Part model, mm, in its own coordinate system. A direction names the side the tool comes from. Give positions to 0.01 mm unless a question says otherwise; leave off trailing zeros. Answer in a Markdown table with one row per item.
from build123d import *

# Parameters (mm, degrees)
BOSS_EXTRUDE1_DEPTH           = 4.7625
SKETCH2_R                     = 4.7625
GEARBOX_WITH_PRESS_FITS_DEPTH = 412.602247496
SKETCH3_R                     = 1.58115
CUT_EXTRUDE1_DEPTH            = 412.602247496
F_4_CLEARANCE_HOLE2_D         = 3.2639
F_4_CLEARANCE_HOLE2_DEPTH     = 28.702
F_4_CLEARANCE_HOLE2_TIP       = 0.980574487
F_4_CLEARANCE_HOLE1_D         = 3.2639
F_4_CLEARANCE_HOLE1_DEPTH     = 4.826
F_4_CLEARANCE_HOLE1_TIP       = 0.980574487
CUT_EXTRUDE2_DEPTH            = 412.602247496


with BuildPart() as part:
    # Sketch1 → Boss-Extrude1 (new body)
    with BuildSketch(Plane(origin=(0, 0, 0), x_dir=(0, 0, -1), z_dir=(1, 0, 0))):
        Polygon((33.297595377, -40.64), (312.697595377, -40.64), (345.995190754, -12.7), (409.563327383, 40.64), (312.697595377, 40.64), (33.297595377, 40.64), (0, 12.7), (-63.568136629, -40.64), align=None)
    extrude(amount=BOSS_EXTRUDE1_DEPTH)

    # Sketch2 → Gearbox (with Press fits) (cut, through all)
    with BuildSketch(Plane(origin=(4.7625, 0, 0), x_dir=(0, 0, -1), z_dir=(1, 0, 0))):
        with Locations((331.004197306, 10)):
            Circle(SKETCH2_R)
    extrude(amount=-GEARBOX_WITH_PRESS_FITS_DEPTH, mode=Mode.SUBTRACT)

    # Sketch3 → Cut-Extrude1 (cut, through all)
    with BuildSketch(Plane(origin=(4.7625, 0, 0), x_dir=(0, 0, -1), z_dir=(1, 0, 0))):
        with Locations((287.297595377, 36.83)):
            Circle(SKETCH3_R)
        with Locations((230.147595377, 36.83)):
            Circle(SKETCH3_R)
        with Locations((172.997595377, 36.83)):
            Circle(SKETCH3_R)
        with Locations((115.847595377, 36.83)):
            Circle(SKETCH3_R)
        with Locations((58.697595377, 36.83)):
            Circle(SKETCH3_R)
        with Locations((58.697595377, -36.83)):
            Circle(SKETCH3_R)
        with Locations((115.847595377, -36.83)):
            Circle(SKETCH3_R)
        with Locations((172.997595377, -36.83)):
            Circle(SKETCH3_R)
        with Locations((230.147595377, -36.83)):
            Circle(SKETCH3_R)
        with Locations((287.297595377, -36.83)):
            Circle(SKETCH3_R)
    extrude(amount=-CUT_EXTRUDE1_DEPTH, mode=Mode.SUBTRACT)

    # #4 Clearance Hole2
    with Locations(Plane(origin=(4.7625, 0, 0), x_dir=(0, 0, -1), z_dir=(1, 0, 0))):
        with Locations((327.962613202, -22.8575274), (342.555759844, -10.612423436), (367.850547356, 10.612423436), (382.443693997, 22.8575274), (18.032577552, 22.8575274), (3.43943091, 10.612423436), (-21.855356602, -10.612423436), (-36.448503243, -22.8575274)):
            Hole(F_4_CLEARANCE_HOLE2_D / 2, depth=F_4_CLEARANCE_HOLE2_DEPTH)
            with Locations((0, 0, -(F_4_CLEARANCE_HOLE2_DEPTH + F_4_CLEARANCE_HOLE2_TIP / 2))):  # 118° drill point
                Cone(0, F_4_CLEARANCE_HOLE2_D / 2, F_4_CLEARANCE_HOLE2_TIP, mode=Mode.SUBTRACT)

    # #4 Clearance Hole1
    with Locations(Plane(origin=(4.7625, 0, 0), x_dir=(0, 0, -1), z_dir=(1, 0, 0))):
        with Locations((198.397595377, 35.56), (198.397595377, -35.56), (198.397595377, 0)):
            Hole(F_4_CLEARANCE_HOLE1_D / 2, depth=F_4_CLEARANCE_HOLE1_DEPTH)
            with Locations((0, 0, -(F_4_CLEARANCE_HOLE1_DEPTH + F_4_CLEARANCE_HOLE1_TIP / 2))):  # 118° drill point
                Cone(0, F_4_CLEARANCE_HOLE1_D / 2, F_4_CLEARANCE_HOLE1_TIP, mode=Mode.SUBTRACT)

    # Sketch11 → Cut-Extrude2 (cut, through all)
    with BuildSketch(Plane(origin=(4.7625, 0, 0), x_dir=(0, 0, -1), z_dir=(1, 0, 0))):
        with BuildLine():
            Line((-21.992783256, -22.332808893), (35.744876514, 26.114840125))
            ThreePointArc((35.744876514, 26.114840125), (37.885826828, 26.856070682), (39.975806034, 25.981383362))
            Line((39.975806034, 25.981383362), (90.827068404, -22.466265655))
            ThreePointArc((90.827068404, -22.466265655), (91.584794367, -25.944437039), (88.636989544, -27.94))
            Line((88.636989544, -27.94), (-19.951932595, -27.94))
            ThreePointArc((-19.951932595, -27.94), (-22.935456666, -25.850913955), (-21.992783256, -22.332808893))
        make_face()
        with BuildLine():
            Line((62.076755313, 22.466265655), (112.793727505, -25.853440749))
            ThreePointArc((112.793727505, -25.853440749), (114.983806365, -26.729706404), (117.173885225, -25.853440749))
            Line((117.173885225, -25.853440749), (167.890857417, 22.466265655))
            ThreePointArc((167.890857417, 22.466265655), (168.648583379, 25.944437039), (165.700778557, 27.94))
            Line((165.700778557, 27.94), (64.266834173, 27.94))
            ThreePointArc((64.266834173, 27.94), (61.31902935, 25.944437039), (62.076755313, 22.466265655))
        make_face()
        with BuildLine():
            Line((186.682516517, 22.828515143), (139.140544325, -22.466265655))
            ThreePointArc((139.140544325, -22.466265655), (138.382818363, -25.944437039), (141.330623185, -27.94))
            Line((141.330623185, -27.94), (188.872595377, -27.94))
            ThreePointArc((188.872595377, -27.94), (191.117659407, -27.01006403), (192.047595377, -24.765))
            Line((192.047595377, -24.765), (192.047595377, 20.529780798))
            ThreePointArc((192.047595377, 20.529780798), (190.123020229, 23.448181506), (186.682516517, 22.828515143))
        make_face()
        with BuildLine():
            Line((204.747595377, 18.932195541), (204.747595377, -24.765))
            ThreePointArc((204.747595377, -24.765), (205.677531347, -27.01006403), (207.922595377, -27.94))
            Line((207.922595377, -27.94), (243.096578394, -27.94))
            ThreePointArc((243.096578394, -27.94), (245.960282851, -26.13606593), (245.569855632, -22.774139707))
            Line((245.569855632, -22.774139707), (210.395872614, 20.923055835))
            ThreePointArc((210.395872614, 20.923055835), (206.867140553, 21.926630398), (204.747595377, 18.932195541))
        make_face()
        with BuildLine():
            Line((225.209113147, 22.774139707), (263.999518653, -25.415794703))
            ThreePointArc((263.999518653, -25.415794703), (266.163859962, -26.584868521), (268.513646551, -25.857125516))
            Line((268.513646551, -25.857125516), (325.94417401, 22.332808893))
            ThreePointArc((325.94417401, 22.332808893), (326.88684742, 25.850913955), (323.903323349, 27.94))
            Line((323.903323349, 27.94), (227.682390385, 27.94))
            ThreePointArc((227.682390385, 27.94), (224.818685928, 26.13606593), (225.209113147, 22.774139707))
        make_face()
    extrude(amount=-CUT_EXTRUDE2_DEPTH, mode=Mode.SUBTRACT)


solid = part.part
(1) Drill centre lines: line 1 along Y through (x, z) = (4.45, 21); line 2 along Y through (x, z) = (4.1, -38.5); line 3 along Y through (x, z) = (0.85, -116.5). Where is each one in solid material? Low to high.
Recorded:
| item | result |
|---|---|
| line 1 | y = -40.64 to -27.76, -21.5 to -12, -9.22 to -4.92 |
| line 2 | y = -40.64 to -27.94, 26.78 to 40.64 |
| line 3 | y = -40.64 to -38.27, -35.39 to -26.34, 27.94 to 35.39, 38.27 to 40.64 |
(2) Saw through at A-A (x = 2.5). Give the number of separate pieces and of enclosed holes in the cut face, plus the area to 3 significant figures.
Recorded:
| item | result |
|---|---|
| separate pieces | 1 |
| enclosed holes | 27 |
| area | 17,700 mm^2 |
(3) Pull direction Y, two halves, no side cores. Call faces 1 (the face through (2.41, -0.98, -244.33)), 2 (the face through (4.762, 10, -170)): +Y half, -Y half, draft (parallel to the pull), parting line (faces both ways), or undercut.
Recorded:
| item | result |
|---|---|
| face 1 | undercut |
| face 2 | draft |
(4) Which spindle directions (+Z, -Z, +X, -X, +Y, -Y) get a long thin tool onto all of the face, cutting with end or side? Do faces 3 (the face through (2.415, 0.498, -163.244)), 4 (the face through (0, 10, -170)). Say none if no direction does.
Recorded:
| item | result |
|---|---|
| face 3 | +X, -X |
| face 4 | +Z, -Z, -X, +Y, -Y |
(5) Pin check, flat tips, straight feed: pin 1 Ø2 at (y, z) = (-22.86, -327.96) entering from +X; pin 2 Ø1.4 at (x, y) = (2.5, 4) entering from +Z; pin 3 Ø1.5 at (x, y) = (2.5, 6.5) entering from +Z. Stop position of each tip, or through.
Recorded:
| item | result |
|---|---|
| pin 1 | passes through |
| pin 2 | stops at z = 11.2 |
| pin 3 | stops at z = 8.28 |
